Geometry: final body of the model. Coordinates: model frame, mm. A direction names the side the tool comes from. Give positions to 0.01 mm unless a question says otherwise; leave off trailing zeros. Loops run counter-clockwise (first coordinate to the right, second up) from the corner with the lowest first, then second, coordinate; pieces in that order, holes last. Notation, with made-up numbers: M 31,-0.75 L 43,-0.75 A26 ccw 43,23.25 Z; hole C -37.5,13 d2. An arc over 180 degrees is marked long. Put each result on its own line as item: value.
```python
from build123d import *

# Parameters (mm, degrees)
SKETCH1_W           = 120
SKETCH1_H           = 55
BOSS_EXTRUDE1_DEPTH = 12.5
SKETCH3_W           = 15.5
SKETCH3_H           = 55
BOSS_EXTRUDE2_DEPTH = 55
SKETCH6_R           = 10
CUT_EXTRUDE1_DEPTH  = 110.001146783
CUT_EXTRUDE4_DEPTH  = 86.914201387
SKETCH8_R           = 4
CUT_EXTRUDE5_DEPTH  = 86.914201387


with BuildPart() as part:
    # Sketch1 → Boss-Extrude1 (new body)
    with BuildSketch(Plane(origin=(0, 0, 0), x_dir=(1, 0, 0), z_dir=(0, 1, 0))):
        Rectangle(SKETCH1_W, SKETCH1_H)
    extrude(amount=-BOSS_EXTRUDE1_DEPTH)

    # Sketch3 → Boss-Extrude2 (add)
    with BuildSketch(Plane(origin=(0, 0, 0), x_dir=(1, 0, 0), z_dir=(0, 1, 0))):
        with Locations((22.25, 0)):
            Rectangle(SKETCH3_W, SKETCH3_H)
        with Locations((-22.25, 0)):
            Rectangle(SKETCH3_W, SKETCH3_H)
    extrude(amount=BOSS_EXTRUDE2_DEPTH)

    # Sketch6 → Cut-Extrude1 (cut, through all)
    with BuildSketch(Plane(origin=(30, 0, 0), x_dir=(0, 0, -1), z_dir=(1, 0, 0))):
        with BuildLine():
            Line((-27.5, 55), (-27.5, 27.5))
            ThreePointArc((-27.5, 27.5), (-19.445436492, 46.945436473), (-2.7e-08, 55))
            Line((-2.7e-08, 55), (-27.5, 55))
        make_face()
        with BuildLine():
            Line((27.5, 55), (-2.7e-08, 55))
            ThreePointArc((-2.7e-08, 55), (19.445436473, 46.945436492), (27.5, 27.5))
            Line((27.5, 27.5), (27.5, 55))
        make_face()
        with Locations((0, 27.5)):
            Circle(SKETCH6_R)
    extrude(amount=-CUT_EXTRUDE1_DEPTH, mode=Mode.SUBTRACT)

    # Sketch7 → Cut-Extrude4 (cut, through all)
    with BuildSketch(Plane(origin=(0, 0, 0), x_dir=(1, 0, 0), z_dir=(0, 1, 0))):
        with BuildLine():
            Line((60, -27.5), (60, -15.5))
            ThreePointArc((60, -15.5), (56.485281374, -23.985281374), (48, -27.5))
            Line((48, -27.5), (60, -27.5))
        make_face()
        with BuildLine():
            ThreePointArc((48, 27.5), (56.485281374, 23.985281374), (60, 15.5))
            Line((60, 15.5), (60, 27.5))
            Line((60, 27.5), (48, 27.5))
        make_face()
        with BuildLine():
            Line((-60, 27.5), (-60, 15.5))
            ThreePointArc((-60, 15.5), (-56.485281374, 23.985281374), (-48, 27.5))
            Line((-48, 27.5), (-60, 27.5))
        make_face()
        with BuildLine():
            ThreePointArc((-48, -27.5), (-56.485281374, -23.985281374), (-60, -15.5))
            Line((-60, -15.5), (-60, -27.5))
            Line((-60, -27.5), (-48, -27.5))
        make_face()
    extrude(amount=-CUT_EXTRUDE4_DEPTH, mode=Mode.SUBTRACT)

    # Sketch8 → Cut-Extrude5 (cut, through all)
    with BuildSketch(Plane(origin=(0, 0, 0), x_dir=(1, 0, 0), z_dir=(0, 1, 0))):
        with Locations(Location((-48, 0, 0), (0, 0, 270))):
            Circle(SKETCH8_R)
        with Locations(Location((48, 0, 0), (0, 0, 270))):
            Circle(SKETCH8_R)
    extrude(amount=-CUT_EXTRUDE5_DEPTH, mode=Mode.SUBTRACT)


solid = part.part
```
Item 1: Line query: probe 1 along X at (y, z) = (-6.5, 0); probe 2 along X at (y, z) = (23, -10.5); probe 3 along Z at (x, y) = (-24, 27). Output: solid intervals per line, ascending. Write a range as [from, to].
Output values:
probe 1: [-60, -52], [-44, 44], [52, 60]
probe 2: [-30, -14.5], [14.5, 30]
probe 3: [-27.5, -9.99], [9.99, 27.5]
Item 2: Mould query, pull axis Y, two halves, no side actions, for faces 5 (the cylindrical face through (22.36, 17.74, 2.17)), 6 (the flat face through (-1, -12.5, 0)), 7 (the cylindrical face through (56.39, -6.16, -24.08)). Classes: pulls with the +Y half, pulls with the -Y half, needs draft (parallel to the pull), parting line crosses it, or undercut.
Output values:
face 5: undercut
face 6: pulls with the -Y half
face 7: needs draft
Item 3: Pin query (flat end, axial travel): pin 1 Ø9 at (x, z) = (-46.5, -8.5) entering from +Y; pin 2 Ø16.5 at (y, z) = (20, 6.5) entering from -X; pin 3 Ø16.5 at (y, z) = (20, -13) entering from +X; pin 4 Ø6.5 at (x, z) = (-48, 0) entering from -Y. Return the tip coordinate at first contact, or that it passes through.
Output values:
pin 1: y = 0
pin 2: x = -30
pin 3: x = 30
pin 4: through
Item 4: Section A-A on y = 22. Output: boundary loops of the cut face in (x, z).
Output values:
outline: M -30,-27.5 L -14.5,-27.5 L -14.5,-8.35 L -30,-8.35 Z; M -30,8.35 L -14.5,8.35 L -14.5,27.5 L -30,27.5 Z; M 14.5,-27.5 L 30,-27.5 L 30,-8.35 L 14.5,-8.35 Z; M 14.5,8.35 L 30,8.35 L 30,27.5 L 14.5,27.5 Z
Item 5: Set-up query: faces 1 (the flat face through (-14.5, 15, 0)), 2 (the flat face through (41, 0, 0)), 3 (the flat face through (-1, -1, 27.5)), 4 (the flat face through (-30, 15, 0)). Return all of +Z, -Z, +X, -X, +Y, -Y with unobstructed straight access to the full face (end or side cutting, diameter ignored); none if empty.
Output values:
face 1: +Z, -Z, +Y
face 2: +Z, -Z, +X, +Y
face 3: +Z, +X, -X, +Y, -Y
face 4: +Z, -Z, -X, +Y
Item 6: Section B-B on x = 22. Output: boundary loops of the cut face in (y, z), then the cut area to 3 significant figures.
Output values:
outline: M -12.5,-27.5 L 27.5,-27.5 A27.5 ccw 27.5,27.5 L -12.5,27.5 Z; hole C 27.5,0 d20
area: 3,070 mm²
